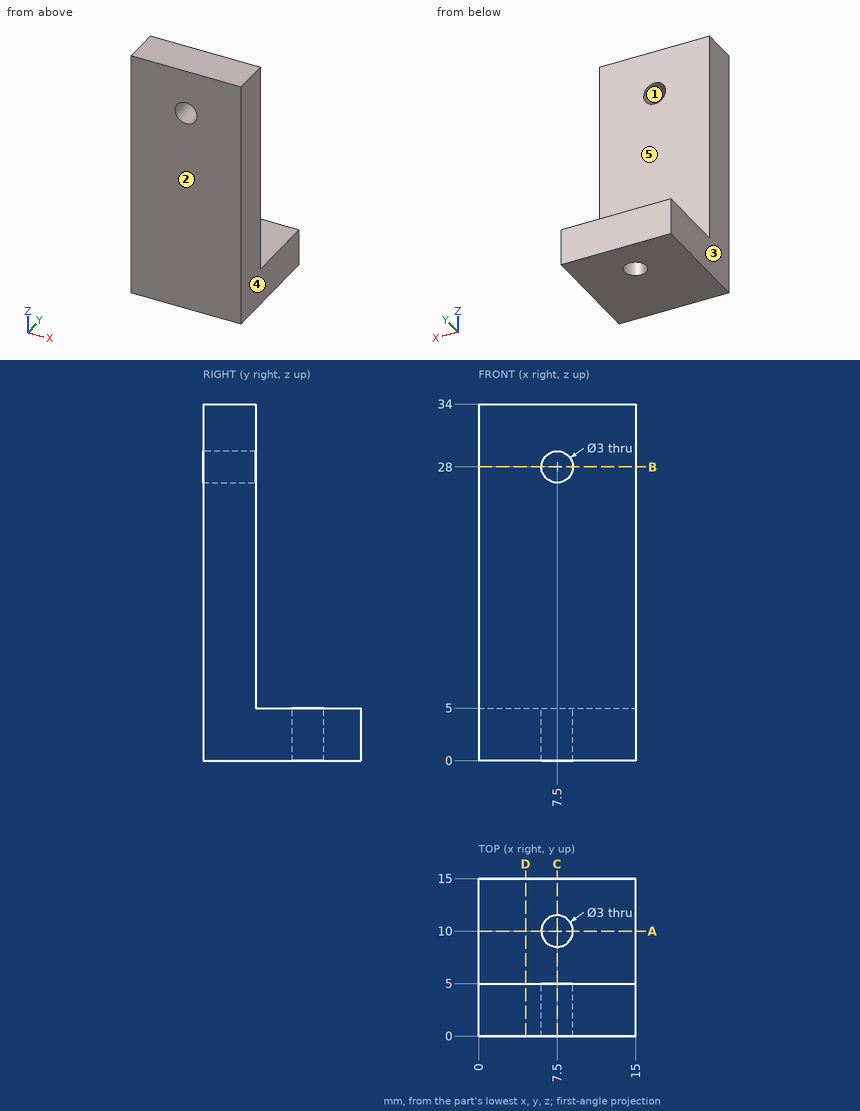
Job drawing, mm, ordinate dimensions from the low corner. One solid piece. A direction names the side the tool comes from. Round coordinates to 2 decimals unless told otherwise and drop trailing zeros. Loops run counter-clockwise (first coordinate to the right, second up) from the corner with the lowest first, then second, coordinate; pieces in that order, holes last. Notation, with made-up numbers: M 44.5,31 L 86.5,31 A21 ccw 86.5,52 Z; hole C 0,10.5 d7. An arc over 180 degrees is marked long. One line per question, with ' | ' between items. Start each with the question number.
Item 1: Cut at D-D, the plane x = 4.5. Write the cut outline in (y, z), plus the area to 3 significant figures.
Item 2: Pin check, flat tips, straight feed: pin 1 Ø2.5 at (x, y) = (7.5, 10) entering from +Z; pin 2 Ø3 at (x, y) = (11, 12) entering from +Z; pin 3 Ø1.5 at (x, z) = (6.5, 25) entering from -Y. Stop position of each tip, or through.
Item 3: Two-plate mould, pull along X, no slides. Class the marked faces 1, 2 and 3: pulls with the +X half, pulls with the -X half, needs draft (parallel to the pull), parting line crosses it, or undercut.
Item 4: Which spindle directions (+Z, -Z, +X, -X, +Y, -Y) get a long thin tool onto all of the face, cutting with end or side? Do the marked faces 4 and 5. Say none if no direction does.
Item 5: Cut at C-C, the plane x = 7.5. Write the cut outline in (y, z), plus the area to 3 significant figures.
Item 6: Cut at A-A, the plane y = 10. Write the cut outline in (x, z), plus the area to 3 significant figures.
Item 7: Wall check: line 1 (X direction, y = 3.75, z = 28); line 2 (Y direction, x = 7.5, z = 1.65); line 3 (Y direction, x = 9, z = 11.5). Give the ranges that are in metal, low to high.
Responses:
1) outline: M 0,0 L 15,0 L 15,5 L 5,5 L 5,34 L 0,34 Z | area: 220 mm²
2) pin 1: passes through | pin 2: stops at z = 5 | pin 3: stops at y = 0
3) face 1: undercut | face 2: needs draft | face 3: pulls with the -X half
4) face 4: +Z, -Z, +X, +Y, -Y | face 5: +Z, +X, -X, +Y
5) outline: M 0,0 L 8.5,0 L 8.5,5 L 5,5 L 5,26.5 L 0,26.5 Z; M 0,29.5 L 5,29.5 L 5,34 L 0,34 Z; M 11.5,0 L 15,0 L 15,5 L 11.5,5 Z | area: 190 mm²
6) outline: M 0,0 L 6,0 L 6,5 L 0,5 Z; M 9,0 L 15,0 L 15,5 L 9,5 Z | area: 60.0 mm²
7) line 1: x = 0 to 6, 9 to 15 | line 2: y = 0 to 8.5, 11.5 to 15 | line 3: y = 0 to 5
